Geometry: final body of the model. Coordinates: model frame, mm. A direction names the side the tool comes from. Coordinates: 2 decimals unless noted, no trailing zeros. Order: outer loops, then holes, each group sorted by start corner. A loop starts at its lowest first (then second) coordinate and runs counter-clockwise, first axis right, second up. Notation, with made-up numbers: (-28, 14.5) -> (30, 14.5) arc R20 cw to (30, 39.5) -> close; hole circle Ø5 at (66.25, 26). An arc over 180 degrees is marked (long way). Answer in a Markdown table with one row per item. Add a question column.
1) Section query A-A on y = 0. Return the cut outline in (x, z), then the cut area to 3 significant figures.
2) Section query B-B on x = 0. Return the cut outline in (y, z), then the cut area to 3 significant figures.
3) Section query C-C on z = 4.5. Return the cut outline in (x, y).
4) Ray query, line 1 (Y direction, x = 2, z = 11); line 2 (Z direction, x = -16.5, y = 10); line 3 (Z direction, x = -2.5, y = -25). Return the intervals inside material, ascending. Write a range as from..to.
5) Set-up query: faces 1 (the face through (26.32, 10.78, 25.67)), 2 (the face through (-21.65, 15.845, 27.335)), 3 (the face through (18.39, 21.7, 25.69)). Return all of +Z, -Z, +X, -X, +Y, -Y with unobstructed straight access to the full face (end or side cutting, diameter ignored); none if empty.
6) Pull-direction query (Y, two-part tool) for faces 4 (the face through (-26.829, 0.093, 27.335)), 5 (the face through (15.49, -21.37, 26.86)), 6 (the face through (8.38, 25.49, 27.33)); classes: +Y half, -Y half, draft (parallel to the pull), parting line (faces both ways), or undercut.
7) Contact query for flat-ended pins moving along their axis: P1, Ø5, axis at x = -24, y = -0.5, coming from the -Z side; P2, Ø6, axis at y = 19, z = -21, coming from the +X side; P3, Ø7, axis at x = -3, y = 1, coming from the +Z side. Output: stop coordinate, or through.
```python
from build123d import *

# Parameters (mm, degrees)
POCKET001_DEPTH    = 335.850526
POLARPATTERN_COUNT = 10


with BuildPart() as part:
    # Sketch003 (on Sketch) → Revolution (revolve)
    with BuildSketch(Plane.YZ):
        Polygon((0, -52.968494), (-18.275258, -52.968494), (-18.275258, 0), (-35.217843, 21.038483), (-18.671614, 33.456837), (-7.212017, 19.226863), (0, 19.226863), align=None)
    revolve(axis=Axis((0, 0, 0), (0, 0, 1)))

    # Sketch004 (on Vertex5 of Revolution) → Pocket001 (cut, through all)
    with BuildSketch(Plane(origin=(0, -5.199434, 24.699477), x_dir=(-1, 0, 0), z_dir=(0, 0.778846, 0.627215))):
        with BuildLine():
            ThreePointArc((2, 14.887447), (0, 14.976512), (-2, 14.887447))
            ThreePointArc((-2, 14.887447), (-3.63932, 19.067787), (-6, 22.887447))
            ThreePointArc((6, 22.887447), (0, 23.473689), (-6, 22.887447))
            ThreePointArc((6, 22.887447), (3.63932, 19.067787), (2, 14.887447))
        make_face()
    pocket001 = extrude(amount=-POCKET001_DEPTH, mode=Mode.SUBTRACT)

    # PolarPattern: Pocket001 ×10 about axis
    polarpattern_axis = Axis((0, 0, 0), (0, 0, 1))
    for i in range(1, POLARPATTERN_COUNT):
        add(pocket001.rotate(polarpattern_axis, i * 360 / POLARPATTERN_COUNT), mode=Mode.SUBTRACT)


solid = part.part
```
Result:
| question | item | result |
|---|---|---|
| 1 | outline | (-35.22, 21.04) -> (-18.28, 0) -> (-18.28, -52.97) -> (18.28, -52.97) -> (18.28, 0) -> (35.22, 21.04) -> (18.67, 33.46) -> (7.21, 19.23) -> (-7.21, 19.23) -> (-18.67, 33.46) -> close |
| 1 | area | 3,360 mm2 |
| 2 | outline | (-34.59, 20.26) -> (-18.28, 0) -> (-18.28, -52.97) -> (18.28, -52.97) -> (18.28, 0) -> (34.59, 20.26) -> (18.49, 33.23) -> (7.21, 19.23) -> (-7.21, 19.23) -> (-18.49, 33.23) -> close |
| 2 | area | 3,340 mm2 |
| 3 | outline | circle Ø43.8 at (0, 0) |
| 4 | line 1 | -27.06..27.06 |
| 4 | line 2 | 1.26..32.99 |
| 4 | line 3 | 8.51..28.61 |
| 5 | face 1 | +Z, +X |
| 5 | face 2 | +Z, -X, +Y |
| 5 | face 3 | +Z, +Y |
| 6 | face 4 | parting line |
| 6 | face 5 | undercut |
| 6 | face 6 | +Y half |
| 7 | P1 | z = 4.01 |
| 7 | P2 | x = 8.83 |
| 7 | P3 | z = 19.23 |
